Part print with two shaded views. Sizes in mm from the minimum x, y, z corner. A direction names the side the tool comes from. Round coordinates to 2 decimals unless told otherwise and drop trailing zeros. Write each loop counter-clockwise with the first axis right and the second up, starting at its lowest first coordinate (ties: lowest second). Pieces come first, ordered by that corner, then holes. Notation, with made-up numbers: (19, 64) -> (69, 64) arc R23 cw to (69, 82) -> close; hole circle Ø7 at (46, 1). An arc over 180 degrees is marked (long way). Return JSON: item names as keys, results as strings. Group by question number.
(1) Drill centre lines: L1, parallel to Y at x = 43, z = 3.9; L2, parallel to Y at x = 23, z = 2.1; L3, parallel to X at y = 12, z = 4.9 (1 decimal). Where is each one in solid material? Low to high. Write a range as from..to.
(2) Drop flat-ended pins along their axis: pin 1 Ø6.5 at (x, y) = (41.5, 10) entering from +Z; pin 2 Ø8.5 at (x, y) = (26.5, 13.5) entering from -Z; pin 3 Ø1.5 at (y, z) = (15.5, 4.5) entering from +X; pin 4 Ø8 at (x, y) = (17, 20) entering from -Z. Give the stop position or say it passes through.
(3) Tool access for the marked faces 4, 5 and 6: list every direction of +Z, -Z, +X, -X, +Y, -Y with a clear straight run to the whole face (end or side of a thin tool).
(4) Mould opens along X. For the marked faces 1, 2 and 3 say: +X half, -X half, draft (parallel to the pull), parting line (faces both ways), or undercut.
(5) Saw through at A-A (z = 3.75). List the corners of the cut face in (x, y) (1 decimal), plus the area to 3 significant figures.
(6) Saw through at C-C (y = 20.75). List the corners of the cut face in (x, z).
(7) Saw through at D-D (x = 24.5). List the corners of the cut face in (y, z).
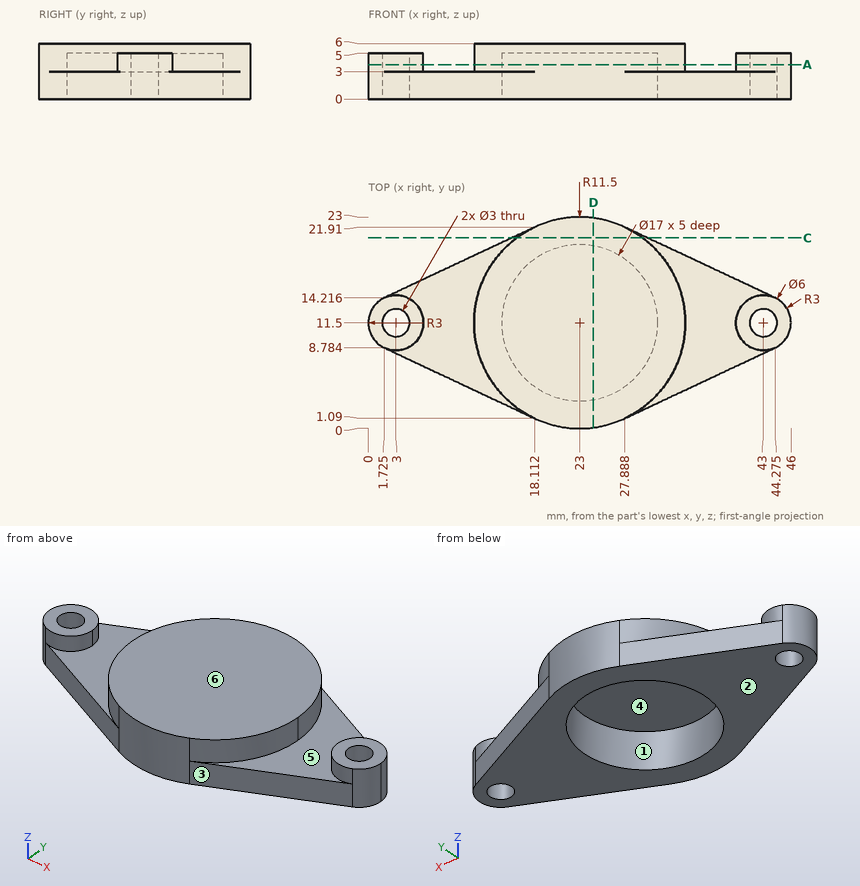
Computed values:
{
 "1": {"L1": "8.5..10, 13..14.5", "L2": "0..3, 20..23", "L3": "0..1.6, 4.4..6, 11.5..14.5, 31.5..34.5, 40..41.6, 44.4..46"},
 "2": {"pin 1": "z = 5", "pin 2": "z = 5", "pin 3": "x = 34.03", "pin 4": "z = 0"},
 "3": {"face 4": "-Z", "face 5": "+Z", "face 6": "+Z, +X, -X, +Y, -Y"},
 "4": {"face 1": "undercut", "face 2": "draft", "face 3": "+X half"},
 "5": {"outline": "circle Ø6 at (3, 11.5); circle Ø23 at (23, 11.5); circle Ø6 at (43, 11.5); hole circle Ø3 at (3, 11.5); hole circle Ø17 at (23, 11.5); hole circle Ø3 at (43, 11.5)", "area": "231 mm2"},
 "6": {"outline": "(15.64, 0) -> (30.36, 0) -> (30.36, 3) -> (29.83, 3) -> (29.83, 6) -> (16.17, 6) -> (16.17, 3) -> (15.64, 3) -> close"},
 "7": {"outline": "(0.1, 0) -> (3.13, 0) -> (3.13, 5) -> (19.87, 5) -> (19.87, 0) -> (22.9, 0) -> (22.9, 6) -> (0.1, 6) -> close"}
}
